```python
from build123d import *

# Parameters (mm, degrees)
SKETCH_W     = 160
SKETCH_H     = 250
PAD_DEPTH    = 18
SKETCH001_W  = 60
SKETCH001_H  = 18
POCKET_DEPTH = 12
CHAMFER_SIZE = 15
FILLET_R     = 10


with BuildPart() as part:
    # Sketch → Pad (new body)
    with BuildSketch(Plane.XY):
        Rectangle(SKETCH_W, SKETCH_H)
    extrude(amount=PAD_DEPTH)

    # Sketch001 → Pocket (cut)
    with BuildSketch(Plane.XY.offset(18)):
        with Locations((0, 51)):
            Rectangle(SKETCH001_W, SKETCH001_H)
    pocket = extrude(amount=-POCKET_DEPTH, mode=Mode.SUBTRACT)

    # Mirrored: Pocket across Sketch001 H_Axis
    add(pocket.mirror(Plane(origin=(0, 0, 18), x_dir=(0, 0, 1), z_dir=(0, 1, 0))), mode=Mode.SUBTRACT)

    # Chamfer
    chamfer_edges = [part.edges().sort_by_distance(p)[0] for p in [
        (-80, -125, 9),
        (-80, 125, 9),
        (80, 125, 9),
        (80, -125, 9),
    ]]
    chamfer(chamfer_edges, length=CHAMFER_SIZE)

    # Fillet
    fillet_edges = [part.edges().sort_by_distance(p)[0] for p in [
        (65, -125, 9),
        (80, -110, 9),
        (-65, -125, 9),
        (-80, -110, 9),
        (-80, 110, 9),
        (-65, 125, 9),
        (65, 125, 9),
        (80, 110, 9),
    ]]
    fillet(fillet_edges, radius=FILLET_R)


solid = part.part
```
Input: part model. Units: mm. Frame: model coordinates. A direction names the side the tool comes from. Give positions to 0.01 mm unless a question says otherwise; leave off trailing zeros. Write each loop counter-clockwise with the first axis right and the second up, starting at its lowest first coordinate (ties: lowest second). Pieces come first, ordered by that corner, then holes. Notation, with made-up numbers: (78.25, 37) - (109.25, 37) arc R26 ccw to (109.25, 56) - close; hole circle Ø4 at (-5, 28). An arc over 180 degrees is marked (long way). Write item = value, one per line. Start each with the question number.
1. Access query for faces 1 (the flat face through (0, 60, 12)), 2 (the cylindrical face through (-64.735, -124.218, 9.126)). Directions: +Z, -Z, +X, -X, +Y, -Y. A direction counts if a zero-diameter tool reaches every point of the face in a straight line with its end or side. Return the directions, or none.
2. Section query C-C, the plane y = 50. Output: boundary loops of the cut face in (x, z), then the cut area to 3 significant figures.
3. Mould query, pull axis X, two halves, no side actions, for faces 3 (the cylindrical face through (-64.735, 124.218, 9.126)), 4 (the flat face through (-1, 125, 9)), 5 (the cylindrical face through (79.218, 109.735, 9.126)), 6 (the flat face through (0, -60, 12)). Classes: released by +X, released by -X, zero draft, split by the parting line, or undercut.
4. Section query B-B, the plane x = -16. Output: boundary loops of the cut face in (y, z), then the cut area to 3 significant figures.
5. First-contact query: pin 1 Ø9 at (x, y) = (-3.5, -51) entering from +Z. Flat tip, straight axial feed; report the tip coordinate or a pass-through.
6. Ray query, L1, parallel to Y at x = 18, z = 9.75; L2, parallel to Z at x = -6.5, y = -50.5; L3, parallel to Y at x = -71.5, z = 11. Return the intervals inside material, ascending.
7. Section query A-A, the plane z = 14.5. Output: boundary loops of the cut face in (x, y).
Check sheet entries:
q1.face_1 = +Z
q1.face_2 = +Z, -Z, -X, -Y
q2.outline = (-80, 0) - (80, 0) - (80, 18) - (30, 18) - (30, 6) - (-30, 6) - (-30, 18) - (-80, 18) - close
q2.area = 2,160 mm2
q3.face_3 = released by -X
q3.face_4 = zero draft
q3.face_5 = released by +X
q3.face_6 = undercut
q4.outline = (-125, 0) - (125, 0) - (125, 18) - (60, 18) - (60, 6) - (42, 6) - (42, 18) - (-42, 18) - (-42, 6) - (-60, 6) - (-60, 18) - (-125, 18) - close
q4.area = 4,070 mm2
q5.pin_1 = 6
q6.L1 = -125 to -60, -42 to 42, 60 to 125
q6.L2 = 0 to 6
q6.L3 = -118.5 to 118.5
q7.outline = (-80, -105.86) arc R10 ccw to (-77.07, -112.93) - (-67.93, -122.07) arc R10 ccw to (-60.86, -125) - (60.86, -125) arc R10 ccw to (67.93, -122.07) - (77.07, -112.93) arc R10 ccw to (80, -105.86) - (80, 105.86) arc R10 ccw to (77.07, 112.93) - (67.93, 122.07) arc R10 ccw to (60.86, 125) - (-60.86, 125) arc R10 ccw to (-67.93, 122.07) - (-77.07, 112.93) arc R10 ccw to (-80, 105.86) - close; hole (-30, -60) - (30, -60) - (30, -42) - (-30, -42) - close; hole (-30, 42) - (30, 42) - (30, 60) - (-30, 60) - close
